Work out the finished part from the listing and answer in its coordinate system (mm). Face numbers are marked on the shaded views. Give positions to 0.01 mm unless a question says otherwise; leave off trailing zeros. Loops run counter-clockwise (first coordinate to the right, second up) from the corner with the lowest first, then second, coordinate; pieces in that order, holes last. Notation, with made-up numbers: (-19, 85) - (-15, 85) arc R10 ccw to (-15, 89) - close; hole circle Ø1 at (-14.5, 41). An arc over 180 degrees is marked (long way). Use CSV: the item, a comma, the result in double quotes.
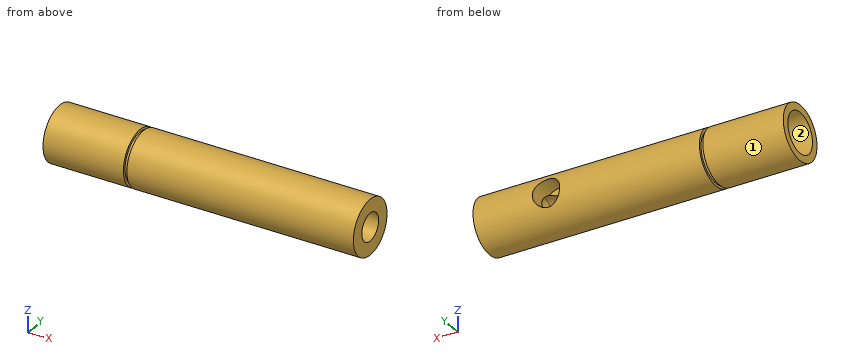
from build123d import *

# Parameters (mm, degrees)
SKETCH2_R          = 4.7625
CUT_EXTRUDE1_DEPTH = 7.62
SKETCH3_W          = 1.1913435
SKETCH3_H          = 1.782578162


with BuildPart() as part:
    # Sketch1 → Revolve1 (revolve)
    with BuildSketch(Plane.XY, mode=Mode.PRIVATE) as revolve1_sk:
        Polygon((53.975, 9.525), (-53.975, 9.525), (-53.975, 6.985), (-35.940357238, 6.985), (-27.793652955, 3.156048987), (29.734276459, 3.156048987), (35.24717222, 4.7625), (53.975, 4.7625), align=None)
    revolve(revolve1_sk.sketch.rotate(Axis((-53.975, 0, 0), (1, 0, 0)), 180), axis=Axis((-53.975, 0, 0), (1, 0, 0)))

    # Sketch2 → Cut-Extrude1 (cut)
    with BuildSketch(Plane(origin=(0, 9.525, 0), x_dir=(1, 0, 0), z_dir=(0, 1, 0))):
        with Locations(Location((28.575, 0, 0), (0, 0, 180))):
            Circle(SKETCH2_R)
    extrude(amount=-CUT_EXTRUDE1_DEPTH, mode=Mode.SUBTRACT)

    # Sketch3 → Cut-Revolve1 (revolve, cut)
    with BuildSketch(Plane(origin=(0, 0, 0), x_dir=(1, 0, 0), z_dir=(0, 1, 0)), mode=Mode.PRIVATE) as cut_revolve1_sk:
        with Locations((-25.4, 9.525)):
            Rectangle(SKETCH3_W, SKETCH3_H)
    revolve(cut_revolve1_sk.sketch.rotate(Axis((-53.975, 0, 0), (1, 0, 0)), 270), axis=Axis((-53.975, 0, 0), (1, 0, 0)), mode=Mode.SUBTRACT)


solid = part.part
Item 1: Find the intervals of material crossed by line 1 (Z direction, x = 40.25, y = 0) (1 decimal); line 2 (X direction, y = -4.25, z = -7.75) (3 decimals); line 3 (X direction, y = 7.75, z = 0) (1 decimal), in increasing order.
Determined:
line 1,"z = -9.5 to -4.8, 4.8 to 9.5"
line 2,"x = -53.975 to -25.996, -24.804 to 53.975"
line 3,"x = -54 to 23.8, 33.3 to 54"
Item 2: A cutting plane is placed at B-B on z = 0. Determine the outline of the cut face in (x, y) (1 decimal).
Determined:
outline,"(-54, -9.5) - (-26, -9.5) - (-26, -8.6) - (-24.8, -8.6) - (-24.8, -9.5) - (54, -9.5) - (54, -4.8) - (35.2, -4.8) - (29.7, -3.2) - (-27.8, -3.2) - (-35.9, -7) - (-54, -7) - close; (-54, 7) - (-35.9, 7) - (-27.8, 3.2) - (23.8, 3.2) - (23.8, 9.5) - (-24.8, 9.5) - (-24.8, 8.6) - (-26, 8.6) - (-26, 9.5) - (-54, 9.5) - close; (33.3, 4.2) - (35.2, 4.8) - (54, 4.8) - (54, 9.5) - (33.3, 9.5) - close"
Item 3: The mould has two halves that part along Z. Classify the marked faces 1 and 2: pulls with the +Z half, pulls with the -Z half, needs draft (parallel to the pull), parting line crosses it, or undercut.
Determined:
face 1,"parting line crosses it"
face 2,"undercut"
Item 4: Given P1, Ø1.5, axis at x = -25.5, z = 2.5, coming from the +Y side; P2, Ø3, axis at x = -27.5, y = 6, coming from the +Z side (3 decimals); P3, Ø1.1, axis at x = 29, z = 3.5, coming from the +Y side (3 decimals); P4, Ø5.5, axis at y = -4.5, z = -3.5, coming from the -X side (3 decimals), each flat-ended and moving along its own axis, determine where each tip first touches the part or whether it passes through.
Determined:
P1,"stops at y = 9.33"
P2,"stops at z = 8.395"
P3,"stops at y = 1.905"
P4,"stops at x = -53.975"
Item 5: A cutting plane is placed at D-D on x = -40. Determine the outline of the cut face in (y, z) (3 decimals), and give its area (3 significant figures).
Determined:
outline,"circle Ø19.05 at (0, 0); hole circle Ø13.97 at (0, 0)"
area,"132 mm²"
Item 6: A cutting plane is placed at A-A on y = 0. Determine the outline of the cut face in (x, z) (1 decimal).
Determined:
outline,"(-54, -9.5) - (-26, -9.5) - (-26, -8.6) - (-24.8, -8.6) - (-24.8, -9.5) - (54, -9.5) - (54, -4.8) - (35.2, -4.8) - (29.7, -3.2) - (-27.8, -3.2) - (-35.9, -7) - (-54, -7) - close; (-54, 7) - (-35.9, 7) - (-27.8, 3.2) - (29.7, 3.2) - (35.2, 4.8) - (54, 4.8) - (54, 9.5) - (-24.8, 9.5) - (-24.8, 8.6) - (-26, 8.6) - (-26, 9.5) - (-54, 9.5) - close"
Item 7: A cutting plane is placed at C-C on x = -22.5. Determine the outline of the cut face in (y, z) (3 decimals).
Determined:
outline,"circle Ø19.05 at (0, 0); hole circle Ø6.312 at (0, 0)"
